Autodesk Inventor part; units mm, degrees
ref_plane "YZ Plane" through (0, 0, 0) normal (1, 0, 0) x (0, 1, 0)
ref_plane "XZ Plane" through (0, 0, 0) normal (0, 1, 0) x (-1, 0, 0)
ref_plane "XY Plane" through (0, 0, 0) normal (0, 0, 1) x (1, 0, 0)
sketch "Boceto1" plane through (0, 0, 0) normal (0, 0, 1) x (1, 0, 0)
  line L0 (-20, 35) -> (20, 35)
  line L1 (20, 35) -> (20, -35)
  line L2 (20, -35) -> (-20, -35)
  line L3 (-20, -35) -> (-20, 35)
  circle A0 centre (0, 20) radius 12.5
  line L4 (-15, -2) -> (15, -2)
  line L5 (15, -2) -> (15, -32)
  line L6 (15, -32) -> (-15, -32)
  line L7 (-15, -32) -> (-15, -2)
  point P0 (0, 0)
  point P1 (0, 35)
  point P2 (-20, 0)
  point P3 (0, -2)
  point P4 (15, -17)
  point P5 (-15, -17)
  dimension "d0" = 70
  dimension "d1" = 25
  dimension "d2" = 20
  dimension "d3" = 40
  dimension "d8" = 30
  dimension "d9" = 30
  dimension "d10" = 3
extrude "Extrusión2" add sketch "Boceto1" along normal blind 10
extrude "Extrusión3" add sketch "Boceto1" along normal blind 162 contours L4 L5 L6 L7
sketch "Boceto2" plane through (-15, -32, 10) normal (0, -1, 0) x (1, 0, 0)
  line L0 (30, 0) -> (0, 0) construction
  line L1 (30, 0) -> (30, 152) construction
  line L2 (0, 152) -> (30, 152) construction
  line L3 (0, 0) -> (0, 152) construction
  line L4 (0, 0) -> (0, 152)
  line L5 (30, 0) -> (30, 152)
  line L6 (0, 152) -> (30, 152)
  line L7 (30, 152) -> (30, 117)
  line L8 (30, 117) -> (0, 117)
  line L9 (0, 117) -> (0, 152)
  point P0 (15, -10)
  point P1 (0, 117)
  dimension "d15" = 35
extrude "Extrusión4" add sketch "Boceto2" along normal blind 9
sketch "Boceto3" plane through (-15, -32, 10) normal (-1, 0, 0) x (0, 0, 1)
  line L0 (117, -9) -> (152, -9)
  circle A0 centre (134.5, -9) radius 25
  point P0 (-10, 32)
  dimension "d18" = 50
extrude "Extrusión5" add sketch "Boceto3" along normal blind 205
properties part number "brazo"
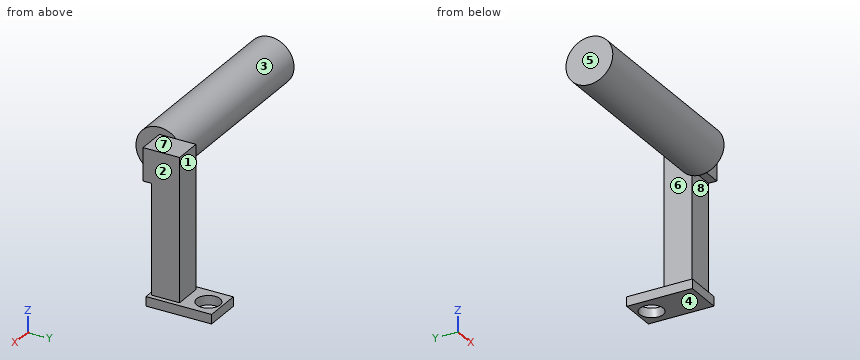
Geometry check sheet. Reference: the model listing, model coordinates, mm. Face numbers are marked on the shaded views. A direction names the side the tool comes from. Coordinates: 2 decimals unless noted, no trailing zeros. Order: outer loops, then holes, each group sorted by start corner. A loop starts at its lowest first (then second) coordinate and runs counter-clockwise, first axis right, second up.
Item 1: Mould release check, pull along Z, two halves, no side actions. Record for the marked faces 5, 6, 7 and 8: released by +Z, released by -Z, zero draft, split by the parting line, or undercut.
Item 2: Section check B-B (x = 0). Enter the section's corners in (y, z).
Item 3: Depth check by flat-ended pin: pin 1 (3 mm diameter, centred on y = 10.5, z = 5, fed in from -X); pin 2 (1.5 mm diameter, centred on x = -87, y = -50.5, fed in from -Z); pin 3 (12 mm diameter, centred on x = -34.5, z = 135.5, fed in from +Y). Enter the tip coordinate at first touch or a pass-through.
Item 4: Section check A-A (y = 20). Enter the section's corners in (x, z).
Item 5: Section check C-C (z = 144.5). Enter the section's corners in (x, y), plus the area to 3 significant figures.
Item 6: Tool access check on the marked faces 1, 2, 3 and 4. Record the directions out of +Z, -Z, +X, -X, +Y, -Y that give a thin tool (end or side, any length) a straight path to the whole face; none if there is none.
Item 7: Section check D-D (y = -18.5). Enter the section's corners in (x, z).
Item 8: Scan lines: line 1 along Y through (x, z) = (0, 5); line 2 along X through (y, z) = (-39, 143); line 3 along X through (y, z) = (-15.5, 73.5). Record each from-to range of solid material in increasing order.
Check sheet entries:
1. face 5: zero draft
1. face 6: undercut
1. face 7: released by +Z
1. face 8: undercut
2. outline: (-41, 127) - (-32, 127) - (-32, 10) - (-35, 10) - (-35, 0) - (7.5, 0) - (7.5, 10) - (-2, 10) - (-2, 162) - (-41, 162) - close; (32.5, 0) - (35, 0) - (35, 10) - (32.5, 10) - close
3. pin 1: stops at x = -20
3. pin 2: stops at z = 121.08
3. pin 3: stops at y = -16.18
4. outline: (-20, 0) - (-12.5, 0) - (-12.5, 10) - (-20, 10) - close; (12.5, 0) - (20, 0) - (20, 10) - (12.5, 10) - close
5. outline: (-220, -66) - (-15, -66) - (-15, -41) - (15, -41) - (15, -2) - (-15, -2) - (-15, -16) - (-220, -16) - close
5. area: 11,400 mm2
6. face 1: +Z, +X, -X, +Y
6. face 2: +Z, +X, +Y, -Y
6. face 3: -X
6. face 4: -Z, +X, -X, +Y, -Y
7. outline: (-220, 133.6) - (-15, 133.6) - (-15, 10) - (-20, 10) - (-20, 0) - (20, 0) - (20, 10) - (15, 10) - (15, 162) - (-15, 162) - (-15, 155.4) - (-220, 155.4) - close
8. line 1: y = -35 to 7.5, 32.5 to 35
8. line 2: x = -220 to 15
8. line 3: x = -15 to 15
